```python
from build123d import *

# Parameters (mm, degrees)
F1_DEPTH = 13
F2_R     = 1.35
F2_R_2   = 1.75
F3_DEPTH = 7.25
F2_R_3   = 2.45
F4_DEPTH = 5.25
F2_R_4   = 3.1
F5_DEPTH = 2.25
F6_W     = 72
F6_H     = 3
F7_DEPTH = 7.25


with BuildPart() as f1:
    # F0 (on Front) → F1 (new body)
    with BuildSketch(Plane.XZ):
        Polygon((0, -4.25), (0, 0), (45, 0), (45, 3), (0, 3), (-27, 3), (-27, -4.25), align=None)
    extrude(amount=F1_DEPTH)

    # F2 (on face) → F3 (cut, through all)
    with BuildSketch(Plane.XY.offset(3)):
        with Locations((-4.75, -6.5)):
            Circle(F2_R)
        with Locations((-22.25, -6.5)):
            Circle(F2_R)
        with Locations((7.485, -6.5)):
            Circle(F2_R_2)
        with Locations((37.515, -6.5)):
            Circle(F2_R_2)
    extrude(amount=-F3_DEPTH, mode=Mode.SUBTRACT)

    # F2 (on face) → F4 (cut, through all)
    with BuildSketch(Plane.XY.offset(3)):
        with Locations((-4.75, -6.5)):
            Circle(F2_R_3)
        with Locations((-4.75, -6.5)):
            Circle(F2_R, mode=Mode.SUBTRACT)
        with Locations((-22.25, -6.5)):
            Circle(F2_R_3)
        with Locations((-22.25, -6.5)):
            Circle(F2_R, mode=Mode.SUBTRACT)
    extrude(amount=-F4_DEPTH, mode=Mode.SUBTRACT)

    # F2 (on face) → F5 (cut, through all)
    with BuildSketch(Plane.XY.offset(3)):
        with Locations((7.485, -6.5)):
            Circle(F2_R_4)
        with Locations((7.485, -6.5)):
            Circle(F2_R_2, mode=Mode.SUBTRACT)
        with Locations((37.515, -6.5)):
            Circle(F2_R_4)
        with Locations((37.515, -6.5)):
            Circle(F2_R_2, mode=Mode.SUBTRACT)
    extrude(amount=-F5_DEPTH, mode=Mode.SUBTRACT)

    # F6 (on face) → F7 (join, through all)
    with BuildSketch(Plane.XY.offset(3)):
        with Locations((9, -14.5)):
            Rectangle(F6_W, F6_H)
        Polygon((45, 0), (45, -13), (45, -16), (48, -16), (48, 0), align=None)
    extrude(amount=-F7_DEPTH)


solid = f1.part
```
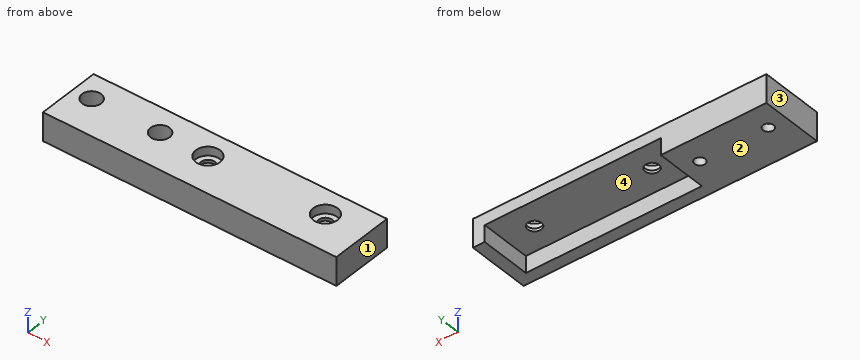
For this review, take the finished solid that the model builds, in its own axes (mm). Face numbers are marked on the shaded views. Coordinates: 2 decimals unless noted, no trailing zeros. Write each loop counter-clockwise with the first axis right and the second up, starting at its lowest first coordinate (ties: lowest second). Pieces come first, ordered by that corner, then holes. Notation, with made-up numbers: (20, 43) -> (72, 43) arc R13 cw to (72, 60) -> close; hole circle Ø10 at (4.5, -31.5). An arc over 180 degrees is marked (long way). Put each result on its own line as item: value.
Q1. Take a section at C-C, the plane y = -6.5. Count the separate pieces of the cut face and the enclosed holes in it, then the cut area to 3 significant figures.
From the geometry:
separate pieces: 5
enclosed holes: 0
area: 257 mm2
Q2. Take a section at D-D, the plane x = 30.5. State the section outline as (y, z) points, then the cut area to 4 significant figures.
From the geometry:
outline: (-16, -4.25) -> (-13, -4.25) -> (-13, 0) -> (0, 0) -> (0, 3) -> (-16, 3) -> close
area: 60.75 mm2
Q3. The part is to be moulded in two halves that separate along X. For the marked faces 1, 2, 3 and 4, say which applies: +X half, -X half, draft (parallel to the pull), parting line (faces both ways), or undercut.
From the geometry:
face 1: +X half
face 2: draft
face 3: -X half
face 4: undercut
Q4. Wall thickness on L1, parallel to X at y = -2, z = -3.25; L2, parallel to X at y = -7.5, z = -2; L3, parallel to X at y = -6, z = 2.5: over which ranges is each line inside the solid? List them lowest first.
From the geometry:
L1: x = -27 to 0, 45 to 48
L2: x = -27 to -24.49, -20.01 to -6.99, -2.51 to 0, 45 to 48
L3: x = -27 to -24.65, -19.85 to -7.15, -2.35 to 4.43, 10.54 to 34.46, 40.57 to 48
Q5. Clearance check with flat-ended pins moving along their axes: pin 1 Ø4 at (x, y) = (27.5, -4.5) entering from -Z; pin 2 Ø1.5 at (x, y) = (38, -8.5) entering from +Z; pin 3 Ø3 at (x, y) = (37.515, -6.5) entering from -Z; pin 4 Ø1.5 at (x, y) = (-5.5, -6) entering from +Z. State where each tip first meets the part, or that it passes through.
From the geometry:
pin 1: stops at z = 0
pin 2: stops at z = 0.75
pin 3: passes through
pin 4: stops at z = -2.25
Q6. Take a section at A-A, the plane x = -22.25. State the section outline as (y, z) points, then the cut area to 3 significant figures.
From the geometry:
outline: (-16, -4.25) -> (-7.85, -4.25) -> (-7.85, -2.25) -> (-8.95, -2.25) -> (-8.95, 3) -> (-16, 3) -> close; (-5.15, -4.25) -> (0, -4.25) -> (0, 3) -> (-4.05, 3) -> (-4.05, -2.25) -> (-5.15, -2.25) -> close
area: 84.9 mm2
Q7. Take a section at B-B, the plane z = -3. State the section outline as (x, y) points, then the cut area to 3 significant figures.
From the geometry:
outline: (-27, -16) -> (48, -16) -> (48, 0) -> (45, 0) -> (45, -13) -> (0, -13) -> (0, 0) -> (-27, 0) -> close; hole circle Ø2.7 at (-22.25, -6.5); hole circle Ø2.7 at (-4.75, -6.5)
area: 604 mm2
